The model under review builds one solid part; all positions refer to its coordinate system, in mm. Face numbers are marked on the shaded views. Coordinates: 2 decimals unless noted, no trailing zeros. Loops run counter-clockwise (first coordinate to the right, second up) from the corner with the lowest first, then second, coordinate; pieces in that order, holes last. Notation, with made-up numbers: M 68.25,11.25 L 80.25,11.25 A28 ccw 80.25,44.25 Z; hole C 77.5,3 d5. An arc over 180 degrees is marked long. Return JSON: item names as keys, results as strings.
```python
from build123d import *

# Parameters (mm, degrees)
F1_DEPTH = 4
F2_R     = 0.75


with BuildPart() as f1:
    # F0 (on Top) → F1 (new body)
    with BuildSketch(Plane.XY):
        with BuildLine():
            ThreePointArc((2.2, 1.8894443628), (0, -2.9), (-2.2, 1.8894443628))
            Line((-2.2, 1.8894443628), (-2.2, 4.4899888641))
            ThreePointArc((-2.2, 4.4899888641), (-3.7064971339, -3.3558723153), (4.25, -2.6339134382))
            ThreePointArc((4.25, -2.6339134382), (3.5, 0), (4.25, 2.6339134382))
            ThreePointArc((4.25, 2.6339134382), (3.3558723153, 3.7064971339), (2.2, 4.4899888641))
            Line((2.2, 4.4899888641), (2.2, 1.8894443628))
        make_face()
        with BuildLine():
            ThreePointArc((4.25, 2.6339134382), (3.5, 0), (4.25, -2.6339134382))
            ThreePointArc((4.25, -2.6339134382), (5, 0), (4.25, 2.6339134382))
        make_face()
        with BuildLine():
            ThreePointArc((4.25, 2.6339134382), (5, 0), (4.25, -2.6339134382))
            ThreePointArc((4.25, -2.6339134382), (8.5, -5), (12.75, -2.6339134382))
            ThreePointArc((12.75, -2.6339134382), (12, 0), (12.75, 2.6339134382))
            ThreePointArc((12.75, 2.6339134382), (11.8558723153, 3.7064971339), (10.7, 4.4899888641))
            Line((10.7, 4.4899888641), (10.7, 1.8894443628))
            ThreePointArc((10.7, 1.8894443628), (8.5, -2.9), (6.3, 1.8894443628))
            Line((6.3, 1.8894443628), (6.3, 4.4899888641))
            ThreePointArc((6.3, 4.4899888641), (5.1441276847, 3.7064971339), (4.25, 2.6339134382))
        make_face()
        with BuildLine():
            ThreePointArc((12.75, 2.6339134382), (12, 0), (12.75, -2.6339134382))
            ThreePointArc((12.75, -2.6339134382), (13.5, 0), (12.75, 2.6339134382))
        make_face()
        with BuildLine():
            ThreePointArc((12.75, 2.6339134382), (13.5, 0), (12.75, -2.6339134382))
            ThreePointArc((12.75, -2.6339134382), (17, -5), (21.25, -2.6339134382))
            ThreePointArc((21.25, -2.6339134382), (20.5, 0), (21.25, 2.6339134382))
            ThreePointArc((21.25, 2.6339134382), (20.3558723153, 3.7064971339), (19.2, 4.4899888641))
            Line((19.2, 4.4899888641), (19.2, 1.8894443628))
            ThreePointArc((19.2, 1.8894443628), (17, -2.9), (14.8, 1.8894443628))
            Line((14.8, 1.8894443628), (14.8, 4.4899888641))
            ThreePointArc((14.8, 4.4899888641), (13.6441276847, 3.7064971339), (12.75, 2.6339134382))
        make_face()
        with BuildLine():
            ThreePointArc((21.25, 2.6339134382), (20.5, 0), (21.25, -2.6339134382))
            ThreePointArc((21.25, -2.6339134382), (22, 0), (21.25, 2.6339134382))
        make_face()
        with BuildLine():
            ThreePointArc((21.25, 2.6339134382), (22, 0), (21.25, -2.6339134382))
            ThreePointArc((21.25, -2.6339134382), (29.2064971339, -3.3558723153), (27.7, 4.4899888641))
            Line((27.7, 4.4899888641), (27.7, 1.8894443628))
            ThreePointArc((27.7, 1.8894443628), (25.5, -2.9), (23.3, 1.8894443628))
            Line((23.3, 1.8894443628), (23.3, 4.4899888641))
            ThreePointArc((23.3, 4.4899888641), (22.1441276847, 3.7064971339), (21.25, 2.6339134382))
        make_face()
    extrude(amount=F1_DEPTH)

    # F2
    f2_edges = [f1.edges().sort_by_distance(p)[0] for p in [
        (-2.2, 4.489989, 2),
        (2.2, 4.489989, 2),
        (6.3, 4.489989, 2),
        (10.7, 4.489989, 2),
        (14.8, 4.489989, 2),
        (19.2, 4.489989, 2),
        (23.3, 4.489989, 2),
        (27.7, 4.489989, 2),
        (21.25, 2.633913, 2),
        (12.75, 2.633913, 2),
        (4.25, 2.633913, 2),
        (21.25, -2.633913, 2),
        (12.75, -2.633913, 2),
        (4.25, -2.633913, 2),
    ]]
    fillet(f2_edges, radius=F2_R)


solid = f1.part
```
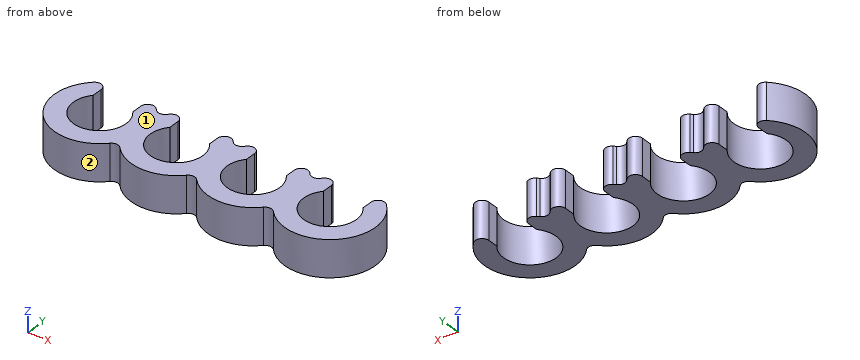
1. Add section C-C on y = 2.5. Give the boundary of the cut face in (x, z), plus the area to 3 significant figures.
Check values:
{"outline": "M -4.33,0 L -2.2,0 L -2.2,4 L -4.33,4 Z; M 2.2,0 L 6.3,0 L 6.3,4 L 2.2,4 Z; M 10.7,0 L 14.8,0 L 14.8,4 L 10.7,4 Z; M 19.2,0 L 23.3,0 L 23.3,4 L 19.2,4 Z; M 27.7,0 L 29.83,0 L 29.83,4 L 27.7,4 Z", "area": "66.2 mm²"}
2. Add section D-D on x = -1. Give the boundary of the cut face in (y, z).
Check values:
{"outline": "M -4.9,0 L -2.72,0 L -2.72,4 L -4.9,4 Z"}
3. Add section B-B on x = 25.5. Give the boundary of the cut face in (y, z), plus the area to 3 significant figures.
Check values:
{"outline": "M -5,0 L -2.9,0 L -2.9,4 L -5,4 Z", "area": "8.40 mm²"}
4. To check wall thickness, follow line 1 (X direction, y = 0, z = 2.1); line 2 (X direction, y = 2, z = 1.4); line 3 (X direction, y = -4, z = 3.25). State the ranges of each line that lie inside material, in increasing order.
Check values:
{"line 1": "-5 to -2.9, 2.9 to 5.6, 11.4 to 14.1, 19.9 to 22.6, 28.4 to 30.5", "line 2": "-4.58 to -2.2, 2.2 to 6.3, 10.7 to 14.8, 19.2 to 23.3, 27.7 to 30.08", "line 3": "-3 to 3, 5.5 to 11.5, 14 to 20, 22.5 to 28.5"}
5. Add section A-A on y = 0. Give the boundary of the cut face in (x, z), plus the area to 3 significant figures.
Check values:
{"outline": "M -5,0 L -2.9,0 L -2.9,4 L -5,4 Z; M 2.9,0 L 5.6,0 L 5.6,4 L 2.9,4 Z; M 11.4,0 L 14.1,0 L 14.1,4 L 11.4,4 Z; M 19.9,0 L 22.6,0 L 22.6,4 L 19.9,4 Z; M 28.4,0 L 30.5,0 L 30.5,4 L 28.4,4 Z", "area": "49.2 mm²"}
6. The part is to be moulded in two halves that separate along X. For the marked faces 1 and 2, say which applies: released by +X, released by -X, zero draft, split by the parting line, or undercut.
Check values:
{"face 1": "zero draft", "face 2": "undercut"}
7. Insertion check: pin 1 Ø0.6 at (y, z) = (2.5, 2) entering from +X; pin 2 Ø1.3 at (y, z) = (2.5, 1) entering from +X; pin 3 Ø0.9 at (y, z) = (2.5, 2.5) entering from -X. Each pin has a flat end and moves straight along its axis. Give the tip position at first contact, or say it passes through.
Check values:
{"pin 1": "x = 29.99", "pin 2": "x = 30.15", "pin 3": "x = -4.56"}
